Check sheet for the modelled part. Datum: model origin and axes. Units: mm. A direction names the side the tool comes from. Round coordinates to 2 decimals unless told otherwise and drop trailing zeros. Write each loop counter-clockwise with the first axis right and the second up, starting at its lowest first coordinate (ties: lowest second). Pieces come first, ordered by that corner, then holes.
Item 1: Depth check by flat-ended pin: pin 1 (1.5 mm diameter, centred on y = 67.5, z = 79.5, fed in from -X). Enter the tip coordinate at first touch or a pass-through.
Item 2: Material ranges on line 1 along Y through (x, z) = (40, 54); line 2 along Z through (x, y) = (46.5, -15.5); line 3 along X through (y, z) = (-24.5, 62.5), recorded low to high.
Item 3: Section check C-C, the plane z = 69. Record the cut outline in (x, y).
Item 4: Section check B-B, the plane x = 31.5. Record the cut outline in (y, z).
Item 5: Section check A-A, the plane y = -14. Record the cut outline in (x, z).
Item 6: Set-up check for faces 1 (the flat face through (54.553, 13, 42)), 2 (the cylindrical face through (-82.982, -44.938, 6.11)), 3 (the flat face through (42, -72.745, 53)): record each of +Z, -Z, +X, -X, +Y, -Y from which the full face is reachable in a straight line by a thin tool's end or side.
Item 7: Release check for a two-part mould opening along Z. For faces 4 (the flat face through (-80.447, 67, 79)), 5 (the flat face through (-16, -1, 85)), 6 (the flat face through (-85.447, -3, 42)), 7 (the flat face through (-80.447, -71, 69)) record: pulls with the +Z half, pulls with the -Z half, needs draft (parallel to the pull), parting line crosses it, or undercut.
Item 8: Section check D-D, the plane z = 53.5. Record the cut outline in (x, y).
from build123d import *

# Parameters (mm, degrees)
F0_W     = 140
F0_H     = 150
F1_DEPTH = 85
F2_W     = 67.2
F2_H     = 40.727277
F3_DEPTH = 25
F4_R     = 2.5
F5_DEPTH = 5


with BuildPart() as f1:
    # F0 (on Top) → F1 (new body)
    with BuildSketch(Plane.XY):
        with Locations((-15.446518, -2.435212)):
            Rectangle(F0_W, F0_H)
    extrude(amount=F1_DEPTH)

    # F2 (on face) → F3 (cut)
    with BuildSketch(Plane.YZ.offset(54.553482)):
        with Locations((-39.144876, 53.109092)):
            Rectangle(F2_W, F2_H)
    extrude(amount=-F3_DEPTH, mode=Mode.SUBTRACT)

    # F4 (on face) → F5 (cut)
    with BuildSketch(Plane(origin=(-85.446518, 0, 0), x_dir=(0, -1, 0), z_dir=(-1, 0, 0))):
        with Locations((-66.875344, 79)):
            Circle(F4_R)
        with Locations((-42.564788, 79)):
            Circle(F4_R)
        with Locations((-66.875344, 16)):
            Circle(F4_R)
        with Locations((-66.875344, 6)):
            Circle(F4_R)
        with Locations((47.435212, 6)):
            Circle(F4_R)
        with Locations((71.435212, 6)):
            Circle(F4_R)
        with Locations((71.435212, 79)):
            Circle(F4_R)
        with Locations((71.435212, 69)):
            Circle(F4_R)
    extrude(amount=-F5_DEPTH, mode=Mode.SUBTRACT)


solid = f1.part
Values found:
1. pin 1: stops at x = -80.45
2. line 1: y = -77.44 to -72.74, -5.54 to 72.56
2. line 2: z = 0 to 32.75, 73.47 to 85
2. line 3: x = -85.45 to 29.55
3. outline: (-85.45, -77.44) - (54.55, -77.44) - (54.55, -72.74) - (29.55, -72.74) - (29.55, -5.54) - (54.55, -5.54) - (54.55, 72.56) - (-85.45, 72.56) - (-85.45, -68.94) - (-80.45, -68.94) - (-80.45, -73.94) - (-85.45, -73.94) - close
4. outline: (-77.44, 0) - (72.56, 0) - (72.56, 85) - (-77.44, 85) - close; hole (-72.74, 32.75) - (-5.54, 32.75) - (-5.54, 73.47) - (-72.74, 73.47) - close
5. outline: (-85.45, 0) - (54.55, 0) - (54.55, 32.75) - (29.55, 32.75) - (29.55, 73.47) - (54.55, 73.47) - (54.55, 85) - (-85.45, 85) - close
6. face 1: +Z, -Z, +X, +Y, -Y
6. face 2: -X
6. face 3: +X
7. face 4: undercut
7. face 5: pulls with the +Z half
7. face 6: needs draft
7. face 7: undercut
8. outline: (-85.45, -77.44) - (54.55, -77.44) - (54.55, -72.74) - (29.55, -72.74) - (29.55, -5.54) - (54.55, -5.54) - (54.55, 72.56) - (-85.45, 72.56) - close
